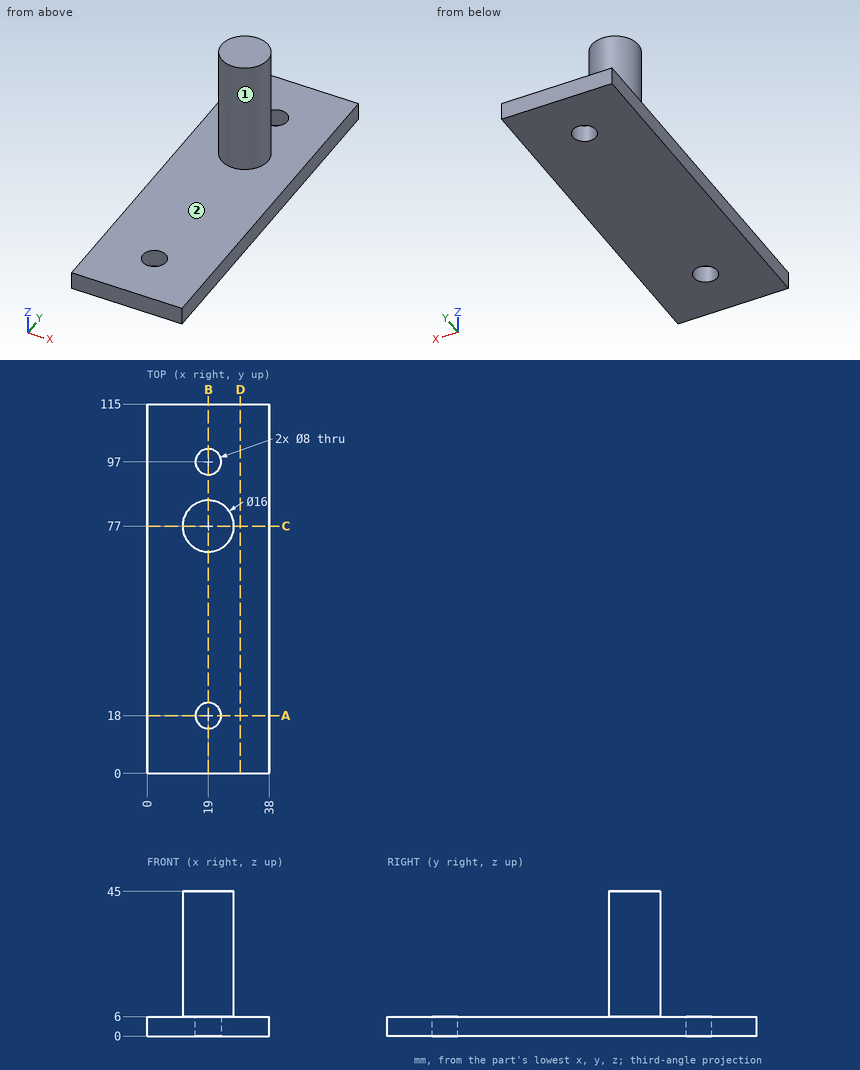
The drawing under review shows one solid part. Ordinate dimensions are in mm from its lowest x, y, z. Give positions to 0.01 mm unless a question says otherwise; leave off trailing zeros. Write each loop counter-clockwise with the first axis right and the second up, starting at its lowest first coordinate (ties: lowest second). Pieces come first, ordered by that corner, then holes. Notation, with made-up numbers: (79.5, -16.5) - (86.5, -16.5) arc R20 ccw to (86.5, -12.5) - close; hole circle Ø4 at (68, 63.25). An arc over 180 degrees is marked (long way). Answer in a Markdown table with one row per item. Add a question column.
1. Draft analysis for pull direction Y (two halves, no side actions). For the marked faces 1 and 2, state which applies: +Y half, -Y half, draft (parallel to the pull), parting line (faces both ways), or undercut.
2. We need section C-C on y = 77. Write out the cut boundary in (x, z).
3. We need section B-B on x = 19. Write out the cut boundary in (y, z), then the cut area to 3 significant figures.
4. Insertion check: P1, Ø5, axis at x = 15, y = 85.5, coming from the +Z side; P2, Ø1.5, axis at x = 30, y = 50, coming from the +Z side; P3, Ø2, axis at y = 85, z = 13, coming from the -X side; P4, Ø10, axis at y = 49, z = 14.5, coming from the +X side. Each pin has a flat end and moves straight along its axis. Give the tip position at first contact, or say it passes through.
5. Wall thickness on line 1 along Y through (x, z) = (19, 3.8); line 2 along Z through (x, y) = (3, 71); line 3 along Y through (x, z) = (25, 13): over which ranges is each line inside the solid? List them lowest first. Write a range as [from, to].
6. We need section D-D on x = 29. Write out the cut boundary in (y, z), then the cut area to 3 significant figures.
7. We need section A-A on y = 18. Write out the cut boundary in (x, z), then the cut area to 3 significant figures.
Ans:
| question | item | result |
|---|---|---|
| 1 | face 1 | parting line |
| 1 | face 2 | draft |
| 2 | outline | (0, 0) - (38, 0) - (38, 6) - (27, 6) - (27, 45) - (11, 45) - (11, 6) - (0, 6) - close |
| 3 | outline | (0, 0) - (14, 0) - (14, 6) - (0, 6) - close; (22, 0) - (93, 0) - (93, 6) - (85, 6) - (85, 45) - (69, 45) - (69, 6) - (22, 6) - close; (101, 0) - (115, 0) - (115, 6) - (101, 6) - close |
| 3 | area | 1,220 mm^2 |
| 4 | P1 | stops at z = 45 |
| 4 | P2 | stops at z = 6 |
| 4 | P3 | stops at x = 15.13 |
| 4 | P4 | passes through |
| 5 | line 1 | y = [0, 14], [22, 93], [101, 115] |
| 5 | line 2 | z = [0, 6] |
| 5 | line 3 | y = [71.71, 82.29] |
| 6 | outline | (0, 0) - (115, 0) - (115, 6) - (0, 6) - close |
| 6 | area | 690 mm^2 |
| 7 | outline | (0, 0) - (15, 0) - (15, 6) - (0, 6) - close; (23, 0) - (38, 0) - (38, 6) - (23, 6) - close |
| 7 | area | 180 mm^2 |
